Design review of the part shown in the three views and the two pictorial views. Dimensions are in mm from the part's minimum x, y and z. A direction names the side the tool comes from. Coordinates: 2 decimals unless noted, no trailing zeros. Loops run counter-clockwise (first coordinate to the right, second up) from the corner with the lowest first, then second, coordinate; pieces in that order, holes last. Notation, with made-up numbers: (39.5, 74.25) -> (96.5, 74.25) arc R15 ccw to (96.5, 96.25) -> close; hole circle Ø1 at (47, 3.5). An arc over 180 degrees is marked (long way). Use CSV: the item, a comma, the result in double quotes.
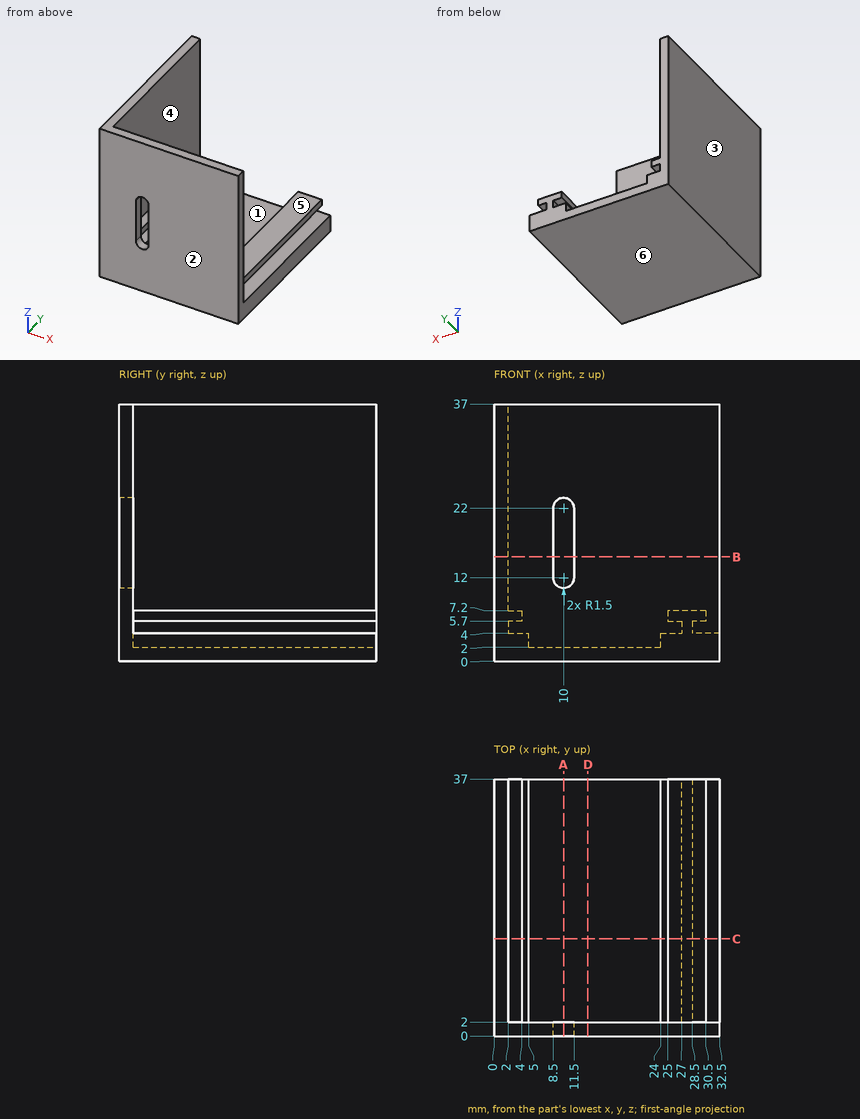
Item 1: Add section C-C (y = 14). Give the boundary of the cut face in (x, z).
Checked values:
outline,"(0, 0) -> (32.5, 0) -> (32.5, 4) -> (28.5, 4) -> (28.5, 5.7) -> (30.5, 5.7) -> (30.5, 7.2) -> (25, 7.2) -> (25, 5.7) -> (27, 5.7) -> (27, 4) -> (24, 4) -> (24, 2) -> (5, 2) -> (5, 4) -> (2, 4) -> (2, 5.7) -> (4, 5.7) -> (4, 7.2) -> (2, 7.2) -> (2, 37) -> (0, 37) -> close"
Item 2: To check wall thickness, follow line 1 along X through (y, z) = (30, 6); line 2 along Z through (x, y) = (25.5, 21); line 3 along X through (y, z) = (19, 30.5). State the ranges of each line that lie inside material, in increasing order.
Checked values:
line 1,"0 to 4, 25 to 30.5"
line 2,"0 to 4, 5.7 to 7.2"
line 3,"0 to 2"
Item 3: Machinability: for the marked faces 5 and 6, which of the approach directions +Z, -Z, +X, -X, +Y, -Y give a long, thin tool a straight path to every point of the face, cutting with its end or side? Answer none if there is none.
Checked values:
face 5,"+Z, +X, +Y"
face 6,"-Z, +X, -X, +Y, -Y"
Item 4: Draft analysis for pull direction X (two halves, no side actions). For the marked faces 1, 2, 3 and 4, state which applies: pulls with the +X half, pulls with the -X half, needs draft (parallel to the pull), parting line crosses it, or undercut.
Checked values:
face 1,"undercut"
face 2,"needs draft"
face 3,"pulls with the -X half"
face 4,"pulls with the +X half"
Item 5: Add section D-D (x = 13.5). Give the boundary of the cut face in (y, z), then the cut area to 3 significant figures.
Checked values:
outline,"(0, 0) -> (37, 0) -> (37, 2) -> (2, 2) -> (2, 37) -> (0, 37) -> close"
area,"144 mm^2"
Item 6: Add section A-A (x = 10). Give the boundary of the cut face in (y, z).
Checked values:
outline,"(0, 0) -> (37, 0) -> (37, 2) -> (2, 2) -> (2, 10.5) -> (0, 10.5) -> close; (0, 23.5) -> (2, 23.5) -> (2, 37) -> (0, 37) -> close"
Item 7: Clearance check with flat-ended pins moving along their axes: pin 1 (1.5 mm diameter, centred on x = 25, y = 24, fed in from +Z); pin 2 (1.5 mm diameter, centred on x = 15.5, y = 6.5, fed in from +Z); pin 3 (0.8 mm diameter, centred on y = 17.5, z = 6.5, fed in from +X). State where each tip first meets the part, or that it passes through.
Checked values:
pin 1,"z = 7.2"
pin 2,"z = 2"
pin 3,"x = 30.5"
Item 8: Add section B-B (z = 15). Give the boundary of the cut face in (x, y), then the cut area to 3 significant figures.
Checked values:
outline,"(0, 0) -> (8.5, 0) -> (8.5, 2) -> (2, 2) -> (2, 37) -> (0, 37) -> close; (11.5, 0) -> (32.5, 0) -> (32.5, 2) -> (11.5, 2) -> close"
area,"129 mm^2"
